from build123d import *

# Parameters (mm, degrees)
F0_R     = 18
F1_DEPTH = 2
F2_R     = 6.5
F3_DEPTH = 3
F4_W     = 46
F4_H     = 8.283501
F5_DEPTH = 25


with BuildPart() as f1:
    # F0 (on Front) → F1 (new body, symmetric)
    with BuildSketch(Plane.XZ):
        Circle(F0_R)
    extrude(amount=F1_DEPTH, both=True)

    # F2 (on face) → F3 (cut)
    with BuildSketch(Plane.XZ.offset(2)):
        Circle(F2_R)
    extrude(amount=-F3_DEPTH, mode=Mode.SUBTRACT)

    # F4 (on face) → F5 (cut)
    with BuildSketch(Plane.XZ.offset(2)):
        with Locations((-4.178571, 14.14175)):
            Rectangle(F4_W, F4_H)
        with Locations((-4.178571, -14.14175)):
            Rectangle(F4_W, F4_H)
    extrude(amount=-F5_DEPTH, mode=Mode.SUBTRACT)


solid = f1.part
Source: CAD feature listing. Evaluate the final solid. Frame: model axes, mm. Give positions to 0.01 mm unless a question says otherwise; leave off trailing zeros. Write each loop counter-clockwise with the first axis right and the second up, starting at its lowest first coordinate (ties: lowest second). Pieces come first, ordered by that corner, then holes. Notation, with made-up numbers: M 37,13.25 L 46,13.25 A20 ccw 46,26.25 Z; hole C -2,47 d11. An arc over 180 degrees is marked long. Return JSON: item names as keys, results as strings. Group by question number.
1) First-contact query: pin 1 Ø1.5 at (y, z) = (-1.5, 7) entering from +X; pin 2 Ø4 at (x, z) = (-0.5, 0.5) entering from -Y; pin 3 Ø1.5 at (y, z) = (1, -8) entering from -X. Flat tips, straight axial feed; report the tip coordinate or a pass-through.
2) Draft query along X for faces 1 (the face through (-5.158, -0.521, -3.955)), 2 (the face through (0, 1, 0)), 3 (the face through (0, 0, 10)), 4 (the face through (-18, 0, 0)). Return one class per face: released by +X, released by -X, zero draft, split by the parting line, or undercut.
3) Cut plane D-D, the plane z = 7. Output: boundary loops of the cut face in (x, y), then the cut area to 3 significant figures.
4) Cut plane B-B, the plane y = 0.45. Output: boundary loops of the cut face in (x, z).
5) Cut plane A-A, the plane x = 0. Output: boundary loops of the cut face in (y, z).
6) Cut plane C-C, the plane z = 0. Output: boundary loops of the cut face in (x, y).
7) Ray query, L1, parallel to Z at x = 0, y = -0.65; L2, parallel to X at y = -0.55, z = -3.75; L3, parallel to X at y = -1.3, z = -4.5. Return the intervals inside material, ascending.
Data:
{
 "1": {"pin 1": "stops at x = 16.88", "pin 2": "stops at y = 1", "pin 3": "stops at x = -16.48"},
 "2": {"face 1": "undercut", "face 2": "undercut", "face 3": "zero draft", "face 4": "released by -X"},
 "3": {"outline": "M -16.58,-2 L 16.58,-2 L 16.58,2 L -16.58,2 Z", "area": "133 mm²"},
 "4": {"outline": "M -14.97,-10 L 14.97,-10 A18 ccw 14.97,10 L -14.97,10 A18 ccw Z; hole C 0,0 d13"},
 "5": {"outline": "M -2,-10 L 2,-10 L 2,10 L -2,10 L -2,6.5 L 1,6.5 L 1,-6.5 L -2,-6.5 Z"},
 "6": {"outline": "M -18,-2 L -6.5,-2 L -6.5,1 L 6.5,1 L 6.5,-2 L 18,-2 L 18,2 L -18,2 Z"},
 "7": {"L1": "z = -10 to -6.5, 6.5 to 10", "L2": "x = -17.61 to -5.31, 5.31 to 17.61", "L3": "x = -17.43 to -4.69, 4.69 to 17.43"}
}
